```python
from build123d import *

# Parameters (mm, degrees)
SKETCH_1_W          = 3
SKETCH_1_H          = 15
EXTRUDE_1_DEPTH     = 3
SKETCH_2_R          = 2.25
CUT_EXTRUDE_1_DEPTH = 10


with BuildPart() as part:
    # 草图1 → 凸台-拉伸1 (new body)
    with BuildSketch(Plane.XY):
        Polygon((2.5, 3), (0, 3), (0, 117), (2.5, 117), (2.5, 120), (17.5, 120), (17.5, 117), (32.5, 117), (32.5, 120), (47.5, 120), (47.5, 117), (62.5, 117), (62.5, 120), (77.5, 120), (77.5, 117), (80, 117), (80, 3), (77.5, 3), (77.5, 0), (62.5, 0), (62.5, 3), (47.5, 3), (47.5, 0), (32.5, 0), (32.5, 3), (17.5, 3), (17.5, 0), (2.5, 0), align=None)
        with Locations((77, 27.5)):
            Rectangle(SKETCH_1_W, SKETCH_1_H, mode=Mode.SUBTRACT)
        with Locations((3, 27.5)):
            Rectangle(SKETCH_1_W, SKETCH_1_H, mode=Mode.SUBTRACT)
    extrude(amount=EXTRUDE_1_DEPTH)

    # 草图2 → 切除-拉伸1 (cut)
    with BuildSketch(Plane.XY.offset(3)):
        with Locations((40, 65)):
            Circle(SKETCH_2_R)
    extrude(amount=-CUT_EXTRUDE_1_DEPTH, mode=Mode.SUBTRACT)


solid = part.part
```
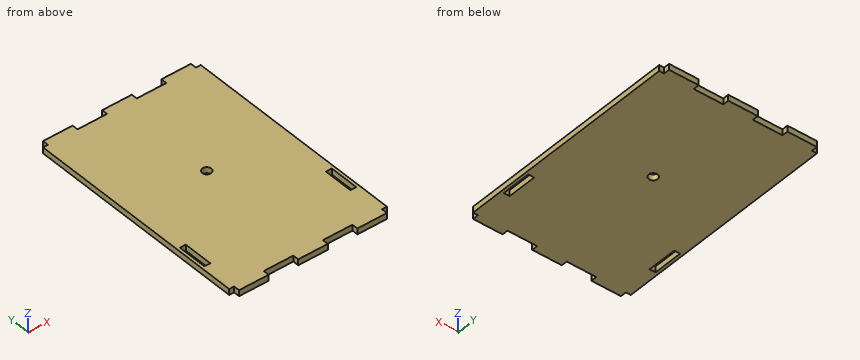
Check sheet for the modelled part. Datum: model origin and axes. Units: mm. Round coordinates to 2 decimals unless told otherwise and drop trailing zeros. Write each loop counter-clockwise with the first axis right and the second up, starting at its lowest first coordinate (ties: lowest second). Pieces come first, ordered by that corner, then holes. Notation, with made-up numbers: M 81,-19 L 98,-19 A21 cw 98,-10 Z; hole C 12.25,16.5 d6. An arc over 180 degrees is marked long. Write item = value, one per line. Start each with the question number.
1. Section check C-C, the plane y = 26. Record the cut outline in (x, z), then the cut area to 3 significant figures.
2. Section check A-A, the plane x = 40. Record the cut outline in (y, z).
3. Section check B-B, the plane y = 65. Record the cut outline in (x, z).
4. Scan lines: line 1 (Y direction, x = 40, z = 1.8); line 2 (Y direction, x = 42, z = 0.45); line 3 (Y direction, x = 21, z = 2.7). Record each from-to range of solid material in increasing order. Write a range as [from, to].
5. Section check D-D, the plane z = 0.6. State how many separate pieces and enclosed holes the cut face has, then the cut area to 3 significant figures.
6. Gauge pin test, flat ends, axial feed: pin 1 (1.5 mm diameter, centred on y = 119, z = 2, fed in from -X); pin 2 (8 mm diameter, centred on x = 33, y = 90, fed in from -Z); pin 3 (0.9 mm diameter, centred on y = 1, z = 2, fed in from +X); pin 4 (1.2 mm diameter, centred on x = 1, z = 1.5, fed in from -Y). Record the tip position at first contact, or that the pin passes through.
Results found:
q1.outline = M 0,0 L 1.5,0 L 1.5,3 L 0,3 Z; M 4.5,0 L 75.5,0 L 75.5,3 L 4.5,3 Z; M 78.5,0 L 80,0 L 80,3 L 78.5,3 Z
q1.area = 222 mm^2
q2.outline = M 0,0 L 62.75,0 L 62.75,3 L 0,3 Z; M 67.25,0 L 120,0 L 120,3 L 67.25,3 Z
q3.outline = M 0,0 L 37.75,0 L 37.75,3 L 0,3 Z; M 42.25,0 L 80,0 L 80,3 L 42.25,3 Z
q4.line_1 = [0, 62.75], [67.25, 120]
q4.line_2 = [0, 63.97], [66.03, 120]
q4.line_3 = [3, 117]
q5.separate_pieces = 1
q5.enclosed_holes = 3
q5.area = 9,280 mm^2
q6.pin_1 = 2.5
q6.pin_2 = 0
q6.pin_3 = 77.5
q6.pin_4 = 3
